from build123d import *

# Parameters (mm, degrees)
F0_R      = 2.5
F1_DEPTH  = 5
F2_W      = 13
F2_H      = 7
F3_DEPTH  = 2.5
F5_DEPTH  = 7
F7_DEPTH  = 7
F8_R      = 1.5
F9_DEPTH  = 5
F10_R     = 1.5
F11_DEPTH = 2.4
F12_R     = 1.5
F13_DEPTH = 5
F14_R     = 1.5
F15_DEPTH = 2.4


with BuildPart() as f1:
    # F0 (on Front) → F1 (new body)
    with BuildSketch(Plane.XZ):
        with BuildLine():
            ThreePointArc((0, 5), (1.464466, 1.464466), (5, 0))
            Line((5, 0), (85, 0))
            ThreePointArc((85, 0), (88.535534, 1.464466), (90, 5))
            Line((90, 5), (90, 57))
            ThreePointArc((90, 57), (88.535534, 60.535534), (85, 62))
            Line((85, 62), (5, 62))
            ThreePointArc((5, 62), (1.464466, 60.535534), (0, 57))
            Line((0, 57), (0, 5))
        make_face()
        with Locations((5.602129, 4.271554)):
            Circle(F0_R, mode=Mode.SUBTRACT)
        with Locations((84.397871, 4.271554)):
            Circle(F0_R, mode=Mode.SUBTRACT)
        with BuildLine():
            Line((3.102129, 55.228446), (3.102129, 57.728446))
            ThreePointArc((3.102129, 57.728446), (5.602129, 60.228446), (8.102129, 57.728446))
            Line((8.102129, 57.728446), (8.102129, 55.228446))
            ThreePointArc((8.102129, 55.228446), (5.602129, 52.728446), (3.102129, 55.228446))
        make_face(mode=Mode.SUBTRACT)
        with BuildLine():
            ThreePointArc((81.897871, 57.728446), (84.397871, 60.228446), (86.897871, 57.728446))
            Line((86.897871, 57.728446), (86.897871, 55.228446))
            ThreePointArc((86.897871, 55.228446), (84.397871, 52.728446), (81.897871, 55.228446))
            Line((81.897871, 55.228446), (81.897871, 57.728446))
        make_face(mode=Mode.SUBTRACT)
    extrude(amount=F1_DEPTH)

    # F2 (on face) → F3 (cut)
    with BuildSketch(Plane.XZ.offset(5)):
        with Locations((6.5, 40.5)):
            Rectangle(F2_W, F2_H)
        with Locations((83.5, 21.5)):
            Rectangle(F2_W, F2_H)
    extrude(amount=-F3_DEPTH, mode=Mode.SUBTRACT)

    # F4 (on face) → F5 (join, through all)
    with BuildSketch(Plane(origin=(0, 0, 44), x_dir=(1, 0, 0), z_dir=(0, 0, -1))):
        Polygon((13, 2.5), (13, 5), (11.25, 2.5), align=None)
        Polygon((7.75, 2.5), (9.25, 2.5), (8.75, 3), (8.25, 3), align=None)
        Polygon((9.75, 2.5), (11.25, 2.5), (10.75, 3), (10.25, 3), align=None)
        Polygon((6.25, 3), (5.75, 2.5), (7.25, 2.5), (6.75, 3), align=None)
        Polygon((4.25, 3), (3.75, 2.5), (5.25, 2.5), (4.75, 3), align=None)
        Polygon((2.25, 3), (1.75, 2.5), (3.25, 2.5), (2.75, 3), align=None)
        Polygon((0.25, 3), (0, 2.5), (1.25, 2.5), (0.75, 3), align=None)
    extrude(amount=F5_DEPTH)

    # F6 (on face) → F7 (join, through all)
    with BuildSketch(Plane.XY.offset(18)):
        Polygon((77, -2.5), (77, -5), (78.75, -2.5), align=None)
        Polygon((80.25, -2.5), (78.75, -2.5), (79.25, -3), (79.75, -3), align=None)
        Polygon((82.25, -2.5), (80.75, -2.5), (81.25, -3), (81.75, -3), align=None)
        Polygon((83.75, -3), (84.25, -2.5), (82.75, -2.5), (83.25, -3), align=None)
        Polygon((85.75, -3), (86.25, -2.5), (84.75, -2.5), (85.25, -3), align=None)
        Polygon((87.75, -3), (88.25, -2.5), (86.75, -2.5), (87.25, -3), align=None)
        Polygon((89.75, -3), (90, -2.5), (88.75, -2.5), (89.25, -3), align=None)
    extrude(amount=F7_DEPTH)

    # F8 (on face) → F9 (cut)
    with BuildSketch(Plane.XZ.offset(5)):
        with Locations((5, 46.5)):
            Circle(F8_R)
        with Locations((5, 34.5)):
            Circle(F8_R)
        with Locations((85, 27.5)):
            Circle(F8_R)
        with Locations((85, 15.5)):
            Circle(F8_R)
    extrude(amount=-F9_DEPTH, mode=Mode.SUBTRACT)

    # F10 (on face) → F11 (cut)
    with BuildSketch(Plane(origin=(0, 0, 0), x_dir=(-1, 0, 0), z_dir=(0, 1, 0))):
        Polygon((-82, 25.767949), (-82, 29.232051), (-85, 30.964102), (-88, 29.232051), (-88, 25.767949), (-85, 24.035898), align=None)
        with Locations((-85, 27.5)):
            Circle(F10_R, mode=Mode.SUBTRACT)
        Polygon((-82, 13.767949), (-82, 17.232051), (-85, 18.964102), (-88, 17.232051), (-88, 13.767949), (-85, 12.035898), align=None)
        with Locations((-85, 15.5)):
            Circle(F10_R, mode=Mode.SUBTRACT)
        Polygon((-8, 36.232051), (-8, 32.767949), (-5, 31.035898), (-2, 32.767949), (-2, 36.232051), (-5, 37.964102), align=None)
        with Locations((-5, 34.5)):
            Circle(F10_R, mode=Mode.SUBTRACT)
        Polygon((-8, 48.232051), (-8, 44.767949), (-5, 43.035898), (-2, 44.767949), (-2, 48.232051), (-5, 49.964102), align=None)
        with Locations((-5, 46.5)):
            Circle(F10_R, mode=Mode.SUBTRACT)
    extrude(amount=-F11_DEPTH, mode=Mode.SUBTRACT)

    # F12 (on face) → F13 (cut)
    with BuildSketch(Plane.XZ.offset(5)):
        with Locations((61, 57)):
            Circle(F12_R)
        with Locations((29, 57)):
            Circle(F12_R)
        with Locations((29, 10)):
            Circle(F12_R)
        with Locations((61, 10)):
            Circle(F12_R)
    extrude(amount=-F13_DEPTH, mode=Mode.SUBTRACT)

    # F14 (on face) → F15 (cut)
    with BuildSketch(Plane(origin=(0, 0, 0), x_dir=(-1, 0, 0), z_dir=(0, 1, 0))):
        Polygon((-58, 8.267949), (-58, 11.732051), (-61, 13.464102), (-64, 11.732051), (-64, 8.267949), (-61, 6.535898), align=None)
        with Locations((-61, 10)):
            Circle(F14_R, mode=Mode.SUBTRACT)
        Polygon((-32, 11.732051), (-32, 8.267949), (-29, 6.535898), (-26, 8.267949), (-26, 11.732051), (-29, 13.464102), align=None)
        with Locations((-29, 10)):
            Circle(F14_R, mode=Mode.SUBTRACT)
    extrude(amount=-F15_DEPTH, mode=Mode.SUBTRACT)


solid = f1.part
CAD build for the part. Positions are in the model's coordinates, mm. A direction names the side the tool comes from. Round coordinates to 2 decimals unless told otherwise and drop trailing zeros. Write each loop counter-clockwise with the first axis right and the second up, starting at its lowest first coordinate (ties: lowest second). Pieces come first, ordered by that corner, then holes. Notation, with made-up numbers: M -25,10.5 L 33,10.5 A30 cw 33,37.5 Z; hole C -27,70.25 d11. An arc over 180 degrees is marked long. Put each result on its own line as item: value. Start each with the question number.
1) Saw through at D-D, the plane y = -1. Count the separate pieces of the cut face and the enclosed holes in it, and give its area (3 significant figures).
2) Saw through at C-C, the plane z = 21.5. Write the cut outline in (x, y).
3) 3-axis set-ups, long thin cutter, end or side, ignore diameter. For faces 5 (the flat face through (86.898, -2, 56)), 6 (the flat face through (83.5, -1.2, 24.9)): which of +Z, -Z, +X, -X, +Y, -Y reach the whole face in a straight line?
4) Pin check, flat tips, straight feed: pin 1 Ø4 at (x, z) = (84.4, 4.27) entering from -Y; pin 2 Ø0.6 at (x, z) = (9.5, 40.5) entering from -Y; pin 3 Ø1.8 at (x, z) = (85.5, 27) entering from +Y; pin 4 Ø1.2 at (x, y) = (86, -3.5) entering from -Z. Stop position of each tip, or through.
5) Saw through at A-A, the plane z = 46.5. Write the cut outline in (x, y).
6) Saw through at B-B, the plane z = 10. Write the cut outline in (x, y).
7) Pull direction X, two halves, no side cores. Call faces 1 (the flat face through (90, -2, 31)), 2 (the flat face through (86, -2.4, 26)), 3 (the cylindrical face through (5.66, -2.46, 52.73)), 4 (the flat face through (44, 0, 31)): pulls with the +X half, pulls with the -X half, needs draft (parallel to the pull), parting line crosses it, or undercut.
8) Drill centre lines: probe 1 along Z at (x, y) = (29, -4); probe 2 along X at (y, z) = (-3.25, 10); probe 3 along Z at (x, y) = (5, -4.35). Where is each one in solid material? Low to high. Write a range as [from, to].
Resolved:
1. separate pieces: 1
1. enclosed holes: 12
1. area: 5,250 mm²
2. outline: M 0,-5 L 77,-5 L 78.75,-2.5 L 79.25,-3 L 79.75,-3 L 80.25,-2.5 L 80.75,-2.5 L 81.25,-3 L 81.75,-3 L 82.25,-2.5 L 82.75,-2.5 L 83.25,-3 L 83.75,-3 L 84.25,-2.5 L 84.75,-2.5 L 85.25,-3 L 85.75,-3 L 86.25,-2.5 L 86.75,-2.5 L 87.25,-3 L 87.75,-3 L 88.25,-2.5 L 88.75,-2.5 L 89.25,-3 L 89.75,-3 L 90,-2.5 L 90,0 L 0,0 Z
3. face 5: +Y, -Y
3. face 6: +Y
4. pin 1: through
4. pin 2: y = -2.55
4. pin 3: y = -2.4
4. pin 4: z = 0.02
5. outline: M 0,-5 L 3.5,-5 L 3.5,-2.4 L 2,-2.4 L 2,0 L 0,0 Z; M 6.5,-5 L 90,-5 L 90,0 L 8,0 L 8,-2.4 L 6.5,-2.4 Z
6. outline: M 0,-5 L 27.5,-5 L 27.5,-2.4 L 26,-2.4 L 26,0 L 0,0 Z; M 30.5,-5 L 59.5,-5 L 59.5,-2.4 L 58,-2.4 L 58,0 L 32,0 L 32,-2.4 L 30.5,-2.4 Z; M 62.5,-5 L 90,-5 L 90,0 L 64,0 L 64,-2.4 L 62.5,-2.4 Z
7. face 1: pulls with the +X half
7. face 2: undercut
7. face 3: undercut
7. face 4: needs draft
8. probe 1: [0, 8.5], [11.5, 55.5], [58.5, 62]
8. probe 2: [0, 27.5], [30.5, 59.5], [62.5, 90]
8. probe 3: [0, 1.85], [6.7, 33], [36, 37], [44, 45], [48, 52.8], [60.15, 62]
